Source: three-view drawing plus pictorial views. Frame: mm from the lowest corner of the part. Coordinates: 2 decimals unless noted, no trailing zeros. Use a Markdown table: item, result. Add a question column.
1. Pin query (flat end, axial travel): pin 1 (2 mm diameter, centred on y = 10, z = 44, fed in from +X) (1 decimal); pin 2 (6.5 mm diameter, centred on x = 9.5, y = 7.5, fed in from +Z) (1 decimal); pin 3 (2 mm diameter, centred on y = 11, z = 21, fed in from -X); pin 4 (1.5 mm diameter, centred on y = 5, z = 7, fed in from +X). Return the tip coordinate at first contact, or that it passes through.
2. Draft query along X for the marked faces 1 and 2. Return one class per face: +X half, -X half, draft (parallel to the pull), parting line (faces both ways), or undercut.
3. Line query: L1, parallel to Z at x = 11, y = 9 (1 decimal); L2, parallel to Y at x = 9, z = 9.5 (1 decimal); L3, parallel to Y at x = 5.75, z = 21. Output: solid intervals per line, ascending. Write a range as [from, to].
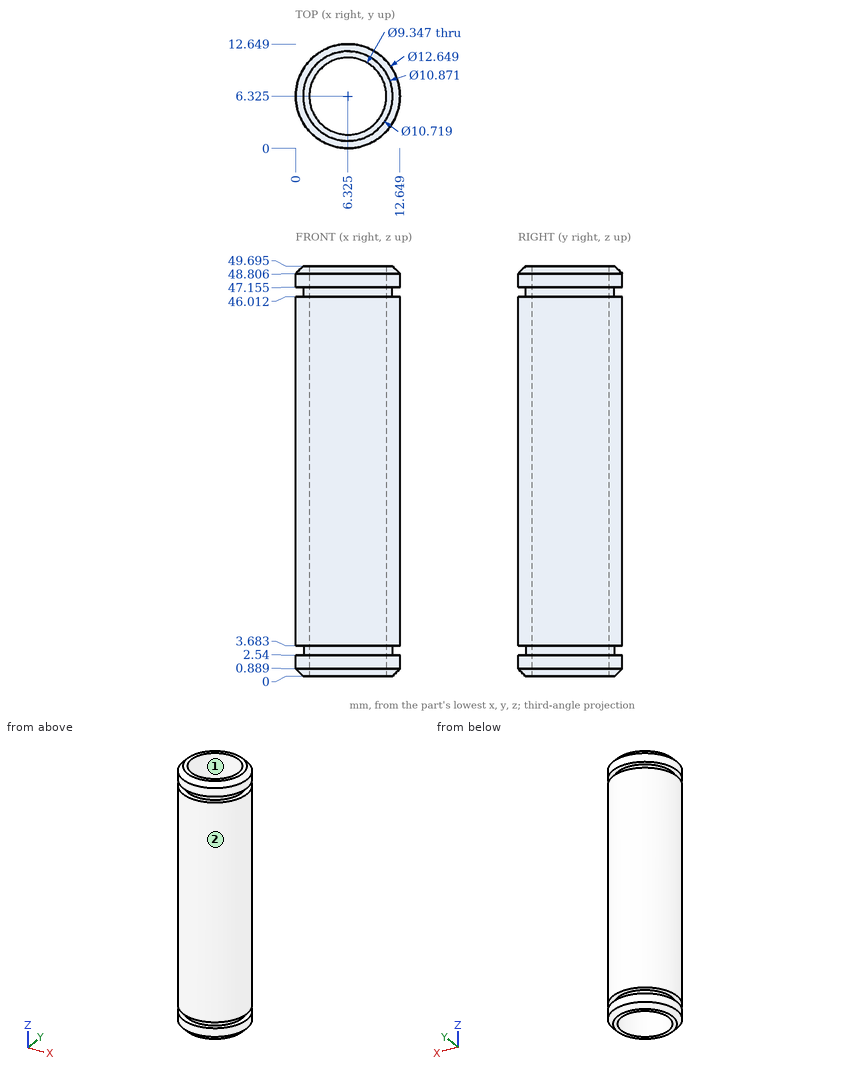
Answers below:
| question | item | result |
|---|---|---|
| 1 | pin 1 | stops at x = 12.1 |
| 1 | pin 2 | stops at z = 49.7 |
| 1 | pin 3 | stops at x = 1.18 |
| 1 | pin 4 | stops at x = 12.62 |
| 2 | face 1 | undercut |
| 2 | face 2 | parting line |
| 3 | L1 | z = [0, 2.5], [3.7, 46], [47.2, 49.7] |
| 3 | L2 | y = [0.6, 2.5], [10.2, 12.1] |
| 3 | L3 | y = [0.03, 1.69], [10.96, 12.62] |
